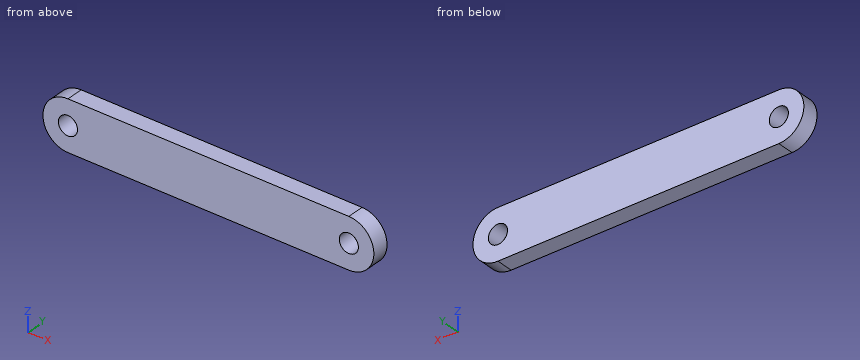
from build123d import *

# Parameters (mm, degrees)
SKETCH1_R           = 1.45
BOSS_EXTRUDE1_DEPTH = 3
SKETCH2_R           = 1.7
CUT_EXTRUDE1_DEPTH  = 55.713846511


with BuildPart() as part:
    # Sketch1 → Boss-Extrude1 (new body)
    with BuildSketch(Plane(origin=(0, 0, 0), x_dir=(1, 0, 0), z_dir=(0, 1, 0))):
        with BuildLine():
            ThreePointArc((0, 4.45), (-4.45, 0), (0, -4.45))
            Line((0, -4.45), (50, -4.45))
            ThreePointArc((50, -4.45), (54.45, 0), (50, 4.45))
            Line((50, 4.45), (0, 4.45))
        make_face()
        with Locations(Location((0, 0, 0), (0, 0, 270))):
            Circle(SKETCH1_R, mode=Mode.SUBTRACT)
        with Locations(Location((50, 0, 0), (0, 0, 270))):
            Circle(SKETCH1_R, mode=Mode.SUBTRACT)
    extrude(amount=BOSS_EXTRUDE1_DEPTH)

    # Sketch2 → Cut-Extrude1 (cut, through all)
    with BuildSketch(Plane(origin=(0, 3, 0), x_dir=(1, 0, 0), z_dir=(0, 1, 0))):
        with Locations(Location((0, 0, 0), (0, 0, 270))):
            Circle(SKETCH2_R)
        with Locations(Location((50, 0, 0), (0, 0, 270))):
            Circle(SKETCH2_R)
    extrude(amount=-CUT_EXTRUDE1_DEPTH, mode=Mode.SUBTRACT)


solid = part.part
Input: part model. Units: mm. Frame: model coordinates. Give positions to 0.01 mm unless a question says otherwise; leave off trailing zeros. Order: outer loops, then holes, each group sorted by start corner. A loop starts at its lowest first (then second) coordinate and runs counter-clockwise, first axis right, second up. Notation, with made-up numbers: (89, -28.5) - (123, -28.5) arc R38 ccw to (123, 9.5) - close; hole circle Ø5 at (-17.75, -4.75). An arc over 180 degrees is marked (long way). Answer as a JSON object with one key per item and string values. Group by question number.
Q1. Cut plane C-C, the plane y = 0.85. Output: boundary loops of the cut face in (x, z), then the cut area to 3 significant figures.
Q2. Cut plane A-A, the plane z = 0. Output: boundary loops of the cut face in (x, y), then the cut area to 3 significant figures.
Q3. Cut plane D-D, the plane z = 2.5. Output: boundary loops of the cut face in (x, y), then the cut area to 3 significant figures.
Q4. Cut plane B-B, the plane x = 49. Output: boundary loops of the cut face in (y, z).
Q5. First-contact query: pin 1 Ø2.5 at (x, z) = (0, 0) entering from +Y; pin 2 Ø1.5 at (x, z) = (47.5, 0.5) entering from -Y. Flat tips, straight axial feed; report the tip coordinate or a pass-through.
Q6. Line query: probe 1 along X at (y, z) = (1, 0); probe 2 along X at (y, z) = (1.1, 1); probe 3 along X at (y, z) = (1.5, 2.25). Output: solid intervals per line, ascending.
Results:
{
 "1": {"outline": "(0, -4.45) - (50, -4.45) arc R4.45 ccw to (50, 4.45) - (0, 4.45) arc R4.45 ccw to start; hole circle Ø3.4 at (0, 0); hole circle Ø3.4 at (50, 0)", "area": "489 mm^2"},
 "2": {"outline": "(-4.45, 0) - (-1.7, 0) - (-1.7, 3) - (-4.45, 3) - close; (1.7, 0) - (48.3, 0) - (48.3, 3) - (1.7, 3) - close; (51.7, 0) - (54.45, 0) - (54.45, 3) - (51.7, 3) - close", "area": "156 mm^2"},
 "3": {"outline": "(-3.68, 0) - (53.68, 0) - (53.68, 3) - (-3.68, 3) - close", "area": "172 mm^2"},
 "4": {"outline": "(0, -4.45) - (3, -4.45) - (3, -1.37) - (0, -1.37) - close; (0, 1.37) - (3, 1.37) - (3, 4.45) - (0, 4.45) - close"},
 "5": {"pin 1": "through", "pin 2": "y = 0"},
 "6": {"probe 1": "-4.45 to -1.7, 1.7 to 48.3, 51.7 to 54.45", "probe 2": "-4.34 to -1.37, 1.37 to 48.63, 51.37 to 54.34", "probe 3": "-3.84 to 53.84"}
}
